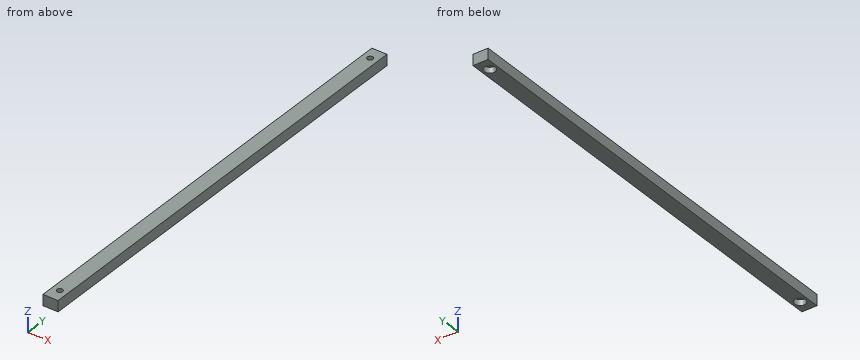
from build123d import *

# Parameters (mm, degrees)
SKETCH_1_W                   = 9
SKETCH_1_H                   = 265
EXTRUDE_1_DEPTH              = 6.5
HOLE_WIZARD_M3_1_D           = 3.4
HOLE_WIZARD_M3_1_DEPTH       = 10.1
HOLE_WIZARD_M3_1_CBORE_D     = 6.5
HOLE_WIZARD_M3_1_CBORE_DEPTH = 3.4
HOLE_WIZARD_M3_1_TIP         = 1.021463052


with BuildPart() as part:
    # 草图1 → 凸台-拉伸1 (new body)
    with BuildSketch(Plane.XY):
        with Locations((4.5, 132.5)):
            Rectangle(SKETCH_1_W, SKETCH_1_H)
    extrude(amount=EXTRUDE_1_DEPTH)

    # M3 六角凹头螺钉的柱形沉头孔1
    with Locations(Plane(origin=(0, 0, 0), x_dir=(-1, 0, 0), z_dir=(0, 0, -1))):
        with Locations((-4.5, 7.5), (-4.5, 257.5)):
            CounterBoreHole(HOLE_WIZARD_M3_1_D / 2, HOLE_WIZARD_M3_1_CBORE_D / 2, HOLE_WIZARD_M3_1_CBORE_DEPTH, depth=HOLE_WIZARD_M3_1_DEPTH)
            with Locations((0, 0, -(HOLE_WIZARD_M3_1_DEPTH + HOLE_WIZARD_M3_1_TIP / 2))):  # 118° drill point
                Cone(0, HOLE_WIZARD_M3_1_D / 2, HOLE_WIZARD_M3_1_TIP, mode=Mode.SUBTRACT)


solid = part.part
Read the model definition and answer for the solid it produces. Units are mm, in the model's axes. Round coordinates to 2 decimals unless told otherwise and drop trailing zeros. Write each loop counter-clockwise with the first axis right and the second up, starting at its lowest first coordinate (ties: lowest second). Pieces come first, ordered by that corner, then holes.
Q1. Find section B-B on z = 1. Determine the outline of the cut face in (x, y).
Values:
outline: (0, 0) - (9, 0) - (9, 265) - (0, 265) - close; hole circle Ø6.5 at (4.5, 7.5); hole circle Ø6.5 at (4.5, 257.5)
Q2. Straight lines are drawn through the part: line 1 (Y direction, x = 4.5, z = 5.45); line 2 (X direction, y = 257.5, z = 2.5); line 3 (X direction, y = 257.5, z = 5.65). For each, find the intervals that lie inside material, in ascending order.
Values:
line 1: y = 0 to 5.8, 9.2 to 255.8, 259.2 to 265
line 2: x = 0 to 1.25, 7.75 to 9
line 3: x = 0 to 2.8, 6.2 to 9
Q3. Find section A-A on x = 4.5. Determine the outline of the cut face in (y, z), and give its area (3 significant figures).
Values:
outline: (0, 0) - (4.25, 0) - (4.25, 3.4) - (5.8, 3.4) - (5.8, 6.5) - (0, 6.5) - close; (9.2, 3.4) - (10.75, 3.4) - (10.75, 0) - (254.25, 0) - (254.25, 3.4) - (255.8, 3.4) - (255.8, 6.5) - (9.2, 6.5) - close; (259.2, 3.4) - (260.75, 3.4) - (260.75, 0) - (265, 0) - (265, 6.5) - (259.2, 6.5) - close
area: 1,660 mm2
Q4. A flat-ended cylindrical pin translates along its axis: P1, Ø5, axis at x = 4.5, y = 257, coming from the -Z side. Find the tip coordinate at first contact, or state that the pin passes through.
Values:
P1: stops at z = 3.4
